Read the model definition and answer for the solid it produces. Units are mm, in the model's axes. A direction names the side the tool comes from. Give positions to 0.01 mm unless a question says otherwise; leave off trailing zeros. Order: outer loops, then holes, each group sorted by start corner. A loop starts at its lowest first (then second) coordinate and runs counter-clockwise, first axis right, second up.
```python
from build123d import *

# Parameters (mm, degrees)
SKETCH1_W           = 25
SKETCH1_H           = 26
SKETCH1_R           = 1.55
BOSS_EXTRUDE1_DEPTH = 1.5
SKETCH2_W           = 1.5
SKETCH2_H           = 26
BOSS_EXTRUDE2_DEPTH = 13.5
SKETCH3_R           = 1.55
CUT_EXTRUDE1_DEPTH  = 13


with BuildPart() as part:
    # Sketch1 → Boss-Extrude1 (new body)
    with BuildSketch(Plane.XY):
        with Locations((8, 0)):
            Rectangle(SKETCH1_W, SKETCH1_H)
        with Locations((0, 10.5)):
            Circle(SKETCH1_R, mode=Mode.SUBTRACT)
        Circle(SKETCH1_R, mode=Mode.SUBTRACT)
        with Locations((0, -10.5)):
            Circle(SKETCH1_R, mode=Mode.SUBTRACT)
    extrude(amount=BOSS_EXTRUDE1_DEPTH)

    # Sketch2 → Boss-Extrude2 (add)
    with BuildSketch(Plane.XY.offset(1.5)):
        with Locations((19.75, 0)):
            Rectangle(SKETCH2_W, SKETCH2_H)
    extrude(amount=BOSS_EXTRUDE2_DEPTH)

    # Sketch3 → Cut-Extrude1 (cut)
    with BuildSketch(Plane(origin=(20.5, 0, 0), x_dir=(0, 0, -1), z_dir=(1, 0, 0))):
        with Locations((-7, 6)):
            Circle(SKETCH3_R)
        with Locations((-7, -6)):
            Circle(SKETCH3_R)
    extrude(amount=-CUT_EXTRUDE1_DEPTH, mode=Mode.SUBTRACT)


solid = part.part
```
1) The part is cut by section A-A on z = 7. Determine the outline of the cut face in (x, y), and give its area (3 significant figures).
Final values:
outline: (19, -13) - (20.5, -13) - (20.5, -7.55) - (19, -7.55) - close; (19, -4.45) - (20.5, -4.45) - (20.5, 4.45) - (19, 4.45) - close; (19, 7.55) - (20.5, 7.55) - (20.5, 13) - (19, 13) - close
area: 29.7 mm2
2) Consider L1, parallel to Y at x = 0, z = 0.65; L2, parallel to Y at x = 19.45, z = 7; L3, parallel to X at y = 4.5, z = 5.5. Determine where each line is inside the solid, lowest interval first.
Final values:
L1: y = -13 to -12.05, -8.95 to -1.55, 1.55 to 8.95, 12.05 to 13
L2: y = -13 to -7.55, -4.45 to 4.45, 7.55 to 13
L3: x = 19 to 20.5
3) The part is cut by section B-B on y = 6. Determine the outline of the cut face in (x, z).
Final values:
outline: (-4.5, 0) - (20.5, 0) - (20.5, 5.45) - (19, 5.45) - (19, 1.5) - (-4.5, 1.5) - close; (19, 8.55) - (20.5, 8.55) - (20.5, 15) - (19, 15) - close
4) The part is cut by section D-D on y = -3.5. Determine the outline of the cut face in (x, z).
Final values:
outline: (-4.5, 0) - (20.5, 0) - (20.5, 15) - (19, 15) - (19, 1.5) - (-4.5, 1.5) - close
5) A tool of negligible diameter and unlimited length cuts with its end or side. For faces 1 (the face through (7, 0, 1.5)), 2 (the face through (20.5, 0, 7)), from which of +Z, -Z, +X, -X, +Y, -Y can it reach the whole face along a straight path? Write none if from no direction.
Final values:
face 1: +Z, -X, +Y, -Y
face 2: +Z, -Z, +X, +Y, -Y
6) For a pull along X with two mould halves and no side action, classify faces 3 (the face through (8, 0, 0)), 4 (the face through (-0.336, -12.013, 0.74)), 5 (the face through (0.715, -1.375, 0.74)), 6 (the face through (-4.5, 0, 1)) as released by +X, released by -X, zero draft, split by the parting line, or undercut.
Final values:
face 3: zero draft
face 4: undercut
face 5: undercut
face 6: released by -X
7) The part is cut by section C-C on x = 0. Determine the outline of the cut face in (y, z).
Final values:
outline: (-13, 0) - (-12.05, 0) - (-12.05, 1.5) - (-13, 1.5) - close; (-8.95, 0) - (-1.55, 0) - (-1.55, 1.5) - (-8.95, 1.5) - close; (1.55, 0) - (8.95, 0) - (8.95, 1.5) - (1.55, 1.5) - close; (12.05, 0) - (13, 0) - (13, 1.5) - (12.05, 1.5) - close
8) Given pin 1 (3 mm diameter, centred on x = 12, y = 5.5, fed in from -Z); pin 2 (4 mm diameter, centred on y = -4, z = 9, fed in from -X); pin 3 (12 mm diameter, centred on x = 3, y = -2.5, fed in from +Z), each flat-ended and moving along its own axis, determine where each tip first touches the part or whether it passes through.
Final values:
pin 1: stops at z = 0
pin 2: stops at x = 19
pin 3: stops at z = 1.5
